from build123d import *

# Parameters (mm, degrees)
F1_DEPTH = 25.4
F3_DEPTH = 38.1
F5_DEPTH = 38.1
F6_SIZE  = 5.08


with BuildPart() as f1:
    # F0 (on Front) → F1 (new body)
    with BuildSketch(Plane.XZ):
        Polygon((-25.4, 0), (0, 0), (0, 482.6), (431.8, 482.6), (431.8, 0), (457.2, 0), (457.2, 508), (-25.4, 508), align=None)
    extrude(amount=-F1_DEPTH)

    # F2 (on face) → F3 (join)
    with BuildSketch(Plane(origin=(0, 0, 0), x_dir=(1, 0, 0), z_dir=(0, 0, -1))):
        with BuildLine():
            Line((-12.7, -12.7), (-12.7, 0))
            ThreePointArc((-12.7, 0), (-21.6802561211, -3.7197438789), (-25.4, -12.7))
            Line((-25.4, -12.7), (-12.7, -12.7))
        make_face()
        with BuildLine():
            ThreePointArc((0, -12.7), (-3.7197438789, -3.7197438789), (-12.7, 0))
            Line((-12.7, 0), (-12.7, -12.7))
            Line((-12.7, -12.7), (0, -12.7))
        make_face()
        with BuildLine():
            Line((-12.7, -25.4), (-12.7, -12.7))
            Line((-12.7, -12.7), (-25.4, -12.7))
            ThreePointArc((-25.4, -12.7), (-21.6802561211, -21.6802561211), (-12.7, -25.4))
        make_face()
        with BuildLine():
            Line((0, -12.7), (-12.7, -12.7))
            Line((-12.7, -12.7), (-12.7, -25.4))
            ThreePointArc((-12.7, -25.4), (-3.7197438789, -21.6802561211), (0, -12.7))
        make_face()
    extrude(amount=F3_DEPTH)

    # F4 (on face) → F5 (join)
    with BuildSketch(Plane(origin=(0, 0, 0), x_dir=(1, 0, 0), z_dir=(0, 0, -1))):
        with BuildLine():
            Line((444.5, -12.7), (431.8, -12.7))
            ThreePointArc((431.8, -12.7), (435.5197438789, -21.6802561211), (444.5, -25.4))
            Line((444.5, -25.4), (444.5, -12.7))
        make_face()
        with BuildLine():
            ThreePointArc((444.5, 0), (435.5197438789, -3.7197438789), (431.8, -12.7))
            Line((431.8, -12.7), (444.5, -12.7))
            Line((444.5, -12.7), (444.5, 0))
        make_face()
        with BuildLine():
            Line((457.2, -12.7), (444.5, -12.7))
            Line((444.5, -12.7), (444.5, -25.4))
            ThreePointArc((444.5, -25.4), (453.4802561211, -21.6802561211), (457.2, -12.7))
        make_face()
        with BuildLine():
            Line((444.5, 0), (444.5, -12.7))
            Line((444.5, -12.7), (457.2, -12.7))
            ThreePointArc((457.2, -12.7), (453.4802561211, -3.7197438789), (444.5, 0))
        make_face()
    extrude(amount=F5_DEPTH)

    # F6
    f6_edges = [f1.edges().sort_by_distance(p)[0] for p in [
        (457.2, 25.4, 254),
        (457.2, 0, 254),
        (-25.4, 25.4, 254),
        (-25.4, 0, 254),
        (215.9, 0, 508),
        (215.9, 25.4, 508),
    ]]
    chamfer(f6_edges, length=F6_SIZE)


solid = f1.part
Design review of the part built by this model. Coordinates are the model's own, in mm. A direction names the side the tool comes from. Coordinates: 2 decimals unless noted, no trailing zeros. Write each loop counter-clockwise with the first axis right and the second up, starting at its lowest first coordinate (ties: lowest second). Pieces come first, ordered by that corner, then holes. Notation, with made-up numbers: (67.5, 26) - (96.5, 26) arc R18 ccw to (96.5, 36) - close; hole circle Ø2 at (16, 22.25). An arc over 180 degrees is marked (long way). One line per item, written item: value.
1) Add section B-B (x = 94). State the section outline as (y, z) points.
Answer sheet:
outline: (0, 482.6) - (25.4, 482.6) - (25.4, 502.92) - (20.32, 508) - (5.08, 508) - (0, 502.92) - close
2) For faces 1 (the face through (454, 22, 0)), 2 (the face through (-22, 3, 0)), 3 (the face through (454, 3, 0)), list the 3-axis set-ups (+Z, -Z, +X, -X, +Y, -Y) from which the entire face can be reached by the end or side of a thin tool; tool diameter is ignored.
Answer sheet:
face 1: -Z, +X, +Y
face 2: -Z, -X, -Y
face 3: -Z, +X, -Y
3) Insertion check: pin 1 (5 mm diameter, centred on x = 284, y = 16.5, fed in from -Z); pin 2 (2 mm diameter, centred on y = 5, z = 370.5, fed in from -X). Each pin has a flat end and moves straight along its axis. Give the tip position at first contact, or say it passes through.
Answer sheet:
pin 1: stops at z = 482.6
pin 2: stops at x = -25.4
4) Add section A-A (z = 146). State the section outline as (x, y) points.
Answer sheet:
outline: (-25.4, 5.08) - (-20.32, 0) - (0, 0) - (0, 25.4) - (-20.32, 25.4) - (-25.4, 20.32) - close; (431.8, 0) - (452.12, 0) - (457.2, 5.08) - (457.2, 20.32) - (452.12, 25.4) - (431.8, 25.4) - close
5) To check wall thickness, follow probe 1 along X at (y, z) = (17, 331); probe 2 along Z at (x, y) = (225, 5); probe 3 along Z at (x, y) = (69, 6.75). State the ranges of each line that lie inside material, in increasing order.
Answer sheet:
probe 1: x = -25.4 to 0, 431.8 to 457.2
probe 2: z = 482.6 to 507.92
probe 3: z = 482.6 to 508
6) Mouldability with a two-part tool opening along X and no side actions: class faces 4 (the face through (0, 13, 238)), 5 (the face through (-25.4, 13, 258)), 6 (the face through (-13, 13, -38.1)), 7 (the face through (-3, 3, 0)) as +X half, -X half, draft (parallel to the pull), parting line (faces both ways), or undercut.
Answer sheet:
face 4: undercut
face 5: -X half
face 6: draft
face 7: undercut
